Can you work these out from the drawing? Everything is in mm from the part's minimum corner. A direction names the side the tool comes from. Round coordinates to 2 decimals unless told otherwise and drop trailing zeros. Write each loop counter-clockwise with the first axis right and the second up, starting at its lowest first coordinate (ties: lowest second). Pieces come first, ordered by that corner, then holes. Notation, with made-up numbers: (-39, 13) -> (-28, 13) arc R29 cw to (-28, 44) -> close; hole circle Ø9 at (17, -3). An arc over 180 degrees is marked (long way). Answer as CSV lines item,"result".
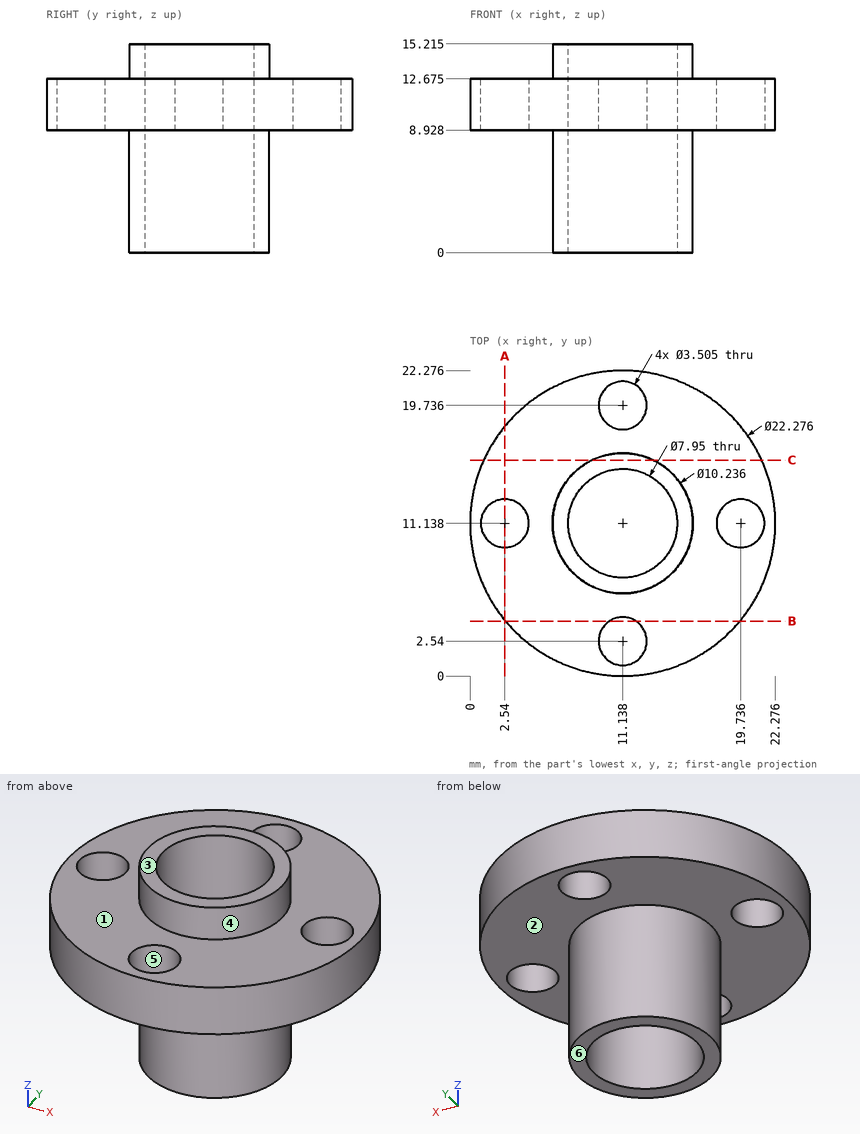
Item 1: I need wall thicknesses on L1, parallel to Y at x = 11.75, z = 10.25 (1 decimal); L2, parallel to Y at x = 11, z = 3.75 (1 decimal); L3, parallel to Z at x = 17, y = 4 (1 decimal). Which ranges of each line are inside material? Lowest first, please.
Results found:
L1,"y = 0 to 0.9, 4.2 to 7.2, 15.1 to 18.1, 21.4 to 22.3"
L2,"y = 6 to 7.2, 15.1 to 16.3"
L3,"z = 8.9 to 12.7"
Item 2: Suppose I cut it at A-A, the plane x = 2.54. List the corners of the cut face in (y, z) for me (1 decimal), then the cut area to 3 significant figures.
Results found:
outline,"(4.1, 8.9) -> (9.4, 8.9) -> (9.4, 12.7) -> (4.1, 12.7) -> close; (12.9, 8.9) -> (18.2, 8.9) -> (18.2, 12.7) -> (12.9, 12.7) -> close"
area,"39.9 mm²"
Item 3: Suppose I cut it at B-B, the plane y = 4. List the corners of the cut face in (x, z) for me (1 decimal), then the cut area to 3 significant figures.
Results found:
outline,"(2.6, 8.9) -> (10.2, 8.9) -> (10.2, 12.7) -> (2.6, 12.7) -> close; (12.1, 8.9) -> (19.7, 8.9) -> (19.7, 12.7) -> (12.1, 12.7) -> close"
area,"56.8 mm²"
Item 4: For the marked faces 1, 2 and 3, which set-ups out of +Z, -Z, +X, -X, +Y, -Y let a thin tool reach every point of the face, with its end or its side?
Results found:
face 1,"+Z"
face 2,"-Z"
face 3,"+Z, +X, -X, +Y, -Y"
Item 5: If we mould it in two halves opening along Y, with no side actions, what happens to the marked faces 4, 5 and 6? For each: pulls with the +Y half, pulls with the -Y half, needs draft (parallel to the pull), parting line crosses it, or undercut.
Results found:
face 4,"parting line crosses it"
face 5,"undercut"
face 6,"needs draft"
Item 6: Suppose I cut it at C-C, the plane y = 15.75. List the corners of the cut face in (x, z) for me (1 decimal).
Results found:
outline,"(1, 8.9) -> (8.9, 8.9) -> (8.9, 0) -> (13.4, 0) -> (13.4, 8.9) -> (21.3, 8.9) -> (21.3, 12.7) -> (13.4, 12.7) -> (13.4, 15.2) -> (8.9, 15.2) -> (8.9, 12.7) -> (1, 12.7) -> close"
Item 7: Will these pins go through, and if not, where does the flat tip stop? pin 1 (5 mm diameter, centred on y = 6.5, z = 2, fed in from +X); pin 2 (5.5 mm diameter, centred on x = 2.54, y = 11.14, fed in from +Z) (1 decimal); pin 3 (2 mm diameter, centred on x = 18.5, y = 3, fed in from -Z).
Results found:
pin 1,"stops at x = 15.79"
pin 2,"stops at z = 12.7"
pin 3,"stops at z = 8.93"
